```python
from build123d import *

# Parameters (mm, degrees)
F1_DEPTH = 7
F2_R     = 2


with BuildPart() as f1:
    # F0 (on Top) → F1 (new body)
    with BuildSketch(Plane.XY):
        with BuildLine():
            ThreePointArc((-10.359665, -4.054993), (-11.124712, 0.080009), (-10.300269, 4.20358))
            ThreePointArc((-10.300269, 4.20358), (-15.677615, 12.123372), (-24.75, 15.178003))
            Line((-24.75, 15.178003), (-24.75, 9.063003))
            Line((-24.75, 9.063003), (-19.620243, 9.063003))
            Line((-19.620243, 9.063003), (-14.490486, 0.178003))
            Line((-14.490486, 0.178003), (-19.620243, -8.706997))
            Line((-19.620243, -8.706997), (-24.75, -8.706997))
            Line((-24.75, -8.706997), (-24.75, -14.821997))
            ThreePointArc((-24.75, -14.821997), (-15.763759, -11.832304), (-10.359665, -4.054993))
        make_face()
        with BuildLine():
            Line((-24.75, 9.063003), (-24.75, 15.178003))
            ThreePointArc((-24.75, 15.178003), (-39.75, 0.178003), (-24.75, -14.821997))
            Line((-24.75, -14.821997), (-24.75, -8.706997))
            Line((-24.75, -8.706997), (-29.879757, -8.706997))
            Line((-29.879757, -8.706997), (-35.009514, 0.178003))
            Line((-35.009514, 0.178003), (-29.879757, 9.063003))
            Line((-29.879757, 9.063003), (-24.75, 9.063003))
        make_face()
        with BuildLine():
            ThreePointArc((-10.300269, 4.20358), (-6.204869, 9.233917), (0, 11.125))
            Line((0, 11.125), (0, 15.178003))
            Line((0, 15.178003), (-24.75, 15.178003))
            ThreePointArc((-24.75, 15.178003), (-15.677615, 12.123372), (-10.300269, 4.20358))
        make_face()
        with BuildLine():
            ThreePointArc((0, 11.125), (6.204869, 9.233917), (10.300269, 4.20358))
            ThreePointArc((10.300269, 4.20358), (15.677615, 12.123372), (24.75, 15.178003))
            Line((24.75, 15.178003), (0, 15.178003))
            Line((0, 15.178003), (0, 11.125))
        make_face()
        with BuildLine():
            Line((0, -14.821997), (0, -11.125))
            ThreePointArc((0, -11.125), (-6.271117, -9.189054), (-10.359665, -4.054993))
            ThreePointArc((-10.359665, -4.054993), (-15.763759, -11.832304), (-24.75, -14.821997))
            Line((-24.75, -14.821997), (0, -14.821997))
        make_face()
        with BuildLine():
            ThreePointArc((24.75, -14.821997), (15.763759, -11.832304), (10.359665, -4.054993))
            ThreePointArc((10.359665, -4.054993), (6.271117, -9.189054), (0, -11.125))
            Line((0, -11.125), (0, -14.821997))
            Line((0, -14.821997), (24.75, -14.821997))
        make_face()
        with BuildLine():
            ThreePointArc((10.300269, 4.20358), (10.91687, 2.141861), (11.125, 0))
            ThreePointArc((11.125, 0), (10.931992, -2.063293), (10.359665, -4.054993))
            ThreePointArc((10.359665, -4.054993), (15.763759, -11.832304), (24.75, -14.821997))
            Line((24.75, -14.821997), (24.75, -8.706997))
            Line((24.75, -8.706997), (19.620243, -8.706997))
            Line((19.620243, -8.706997), (14.490486, 0.178003))
            Line((14.490486, 0.178003), (19.620243, 9.063003))
            Line((19.620243, 9.063003), (24.75, 9.063003))
            Line((24.75, 9.063003), (24.75, 15.178003))
            ThreePointArc((24.75, 15.178003), (15.677615, 12.123372), (10.300269, 4.20358))
        make_face()
        with BuildLine():
            ThreePointArc((39.75, 0.178003), (35.356602, 10.784605), (24.75, 15.178003))
            Line((24.75, 15.178003), (24.75, 9.063003))
            Line((24.75, 9.063003), (29.879757, 9.063003))
            Line((29.879757, 9.063003), (35.009514, 0.178003))
            Line((35.009514, 0.178003), (29.879757, -8.706997))
            Line((29.879757, -8.706997), (24.75, -8.706997))
            Line((24.75, -8.706997), (24.75, -14.821997))
            ThreePointArc((24.75, -14.821997), (35.356602, -10.428599), (39.75, 0.178003))
        make_face()
    extrude(amount=F1_DEPTH)

    # F2
    f2_edges = [f1.edges().sort_by_distance(p)[0] for p in [
        (0, 15.178003, 7),
        (0, 15.178003, 0),
    ]]
    fillet(f2_edges, radius=F2_R)


solid = f1.part
```
The model under review builds one solid part; all positions refer to its coordinate system, in mm. A direction names the side the tool comes from. Round coordinates to 2 decimals unless told otherwise and drop trailing zeros. Loops run counter-clockwise (first coordinate to the right, second up) from the corner with the lowest first, then second, coordinate; pieces in that order, holes last. Notation, with made-up numbers: (62.5, -40) -> (109.5, -40) arc R18 ccw to (109.5, -21) -> close; hole circle Ø6 at (-26.75, 41). An arc over 180 degrees is marked (long way). Answer as a JSON object with one key per item and string values. Group by question number.
1) For pin 1 Ø3.5 at (x, z) = (25.5, 4) entering from +Y; pin 2 Ø1.5 at (y, z) = (-3, 5.5) entering from -X, all flat-tipped, find the tip position at first contact; note any pin that passes through.
2) We need section B-B on x = -12. Write out the cut boundary in (y, z), then the cut area to 3 significant figures.
3) For faces 1 (the face through (-9, 9, 7)), 2 (the face through (10.91, 2.17, 3.45)), list the 3-axis set-ups (+Z, -Z, +X, -X, +Y, -Y) from which the entire face can be reached by the end or side of a thin tool; tool diameter is ignored.
4) For line 1 (X direction, y = -4, z = 2.75); line 2 (X direction, y = 4.5, z = 1); line 3 (Y direction, x = 29.5, z = 4.5), list the stretches that pass through material, from the lowest coordinate up. Write a range as [from, to].
5) We need section D-D on y = 1. Give the number of separate pieces and of enclosed holes in the cut face, then the cut area to 3 significant figures.
6) We need section C-C on x = 18. Write out the cut boundary in (y, z), then the cut area to 3 significant figures.
7) Mouldability with a two-part tool opening along Y and no side actions: class faces 3 (the face through (-0.346, 14.608, 6.399)), 4 (the face through (-25, 9.063, 3)), 5 (the face through (-39.746, 0.508, 3.479)) as released by +Y, released by -Y, zero draft, split by the parting line, or undercut.
8) We need section A-A on z = 4. Write out the cut boundary in (x, y) (3 decimals).
Result set:
{
 "1": {"pin 1": "y = 15.18", "pin 2": "x = -39.53"},
 "2": {"outline": "(-14.82, 2) arc R2 ccw to (-12.82, 0) -> (13.18, 0) arc R2 ccw to (15.18, 2) -> (15.18, 5) arc R2 ccw to (13.18, 7) -> (-12.82, 7) arc R2 ccw to (-14.82, 5) -> close", "area": "207 mm²"},
 "3": {"face 1": "+Z, +X, -X, +Y, -Y", "face 2": "+Z, -Z"},
 "4": {"line 1": "[-39.16, -32.6], [-16.9, -10.38], [10.38, 16.9], [32.6, 39.16]", "line 2": "[-38.83, -32.51], [-16.99, -10.17], [10.17, 16.99], [32.51, 38.83]", "line 3": "[-14.05, -8.71], [9.06, 14.41]"},
 "5": {"separate pieces": "4", "enclosed holes": "0", "area": "124 mm²"},
 "6": {"outline": "(-14.82, 2) arc R2 ccw to (-12.82, 0) -> (-5.9, 0) -> (-5.9, 7) -> (-12.82, 7) arc R2 ccw to (-14.82, 5) -> close; (6.26, 0) -> (13.18, 0) arc R2 ccw to (15.18, 2) -> (15.18, 5) arc R2 ccw to (13.18, 7) -> (6.26, 7) -> close", "area": "121 mm²"},
 "7": {"face 3": "released by +Y", "face 4": "undercut", "face 5": "split by the parting line"},
 "8": {"outline": "(-24.75, -14.822) -> (24.75, -14.822) arc R15 ccw to (39.75, 0.178) arc R15 ccw to (24.75, 15.178) -> (-24.75, 15.178) arc R15 ccw to start; hole (-35.01, 0.178) -> (-29.88, -8.707) -> (-19.62, -8.707) -> (-14.49, 0.178) -> (-19.62, 9.063) -> (-29.88, 9.063) -> close; hole (-10.36, -4.055) arc R11.125 ccw to (0, -11.125) arc R11.125 ccw to (10.36, -4.055) arc R11.125 ccw to (11.125, 0) arc R11.125 ccw to (10.3, 4.204) arc R11.125 ccw to (-10.3, 4.204) arc R11.125 ccw to start; hole (14.49, 0.178) -> (19.62, -8.707) -> (29.88, -8.707) -> (35.01, 0.178) -> (29.88, 9.063) -> (19.62, 9.063) -> close"}
}
